Drawing for the job (mm, zero at the part's lowest x, y, z). Coordinates: 2 decimals unless noted, no trailing zeros. Loops run counter-clockwise (first coordinate to the right, second up) from the corner with the lowest first, then second, coordinate; pieces in that order, holes last. Notation, with made-up numbers: (-23, -39.5) - (25, -39.5) arc R15 cw to (25, -23.5) - close; hole circle Ø3 at (-2.5, -12). An arc over 180 degrees is marked (long way). One line per item, written item: value.
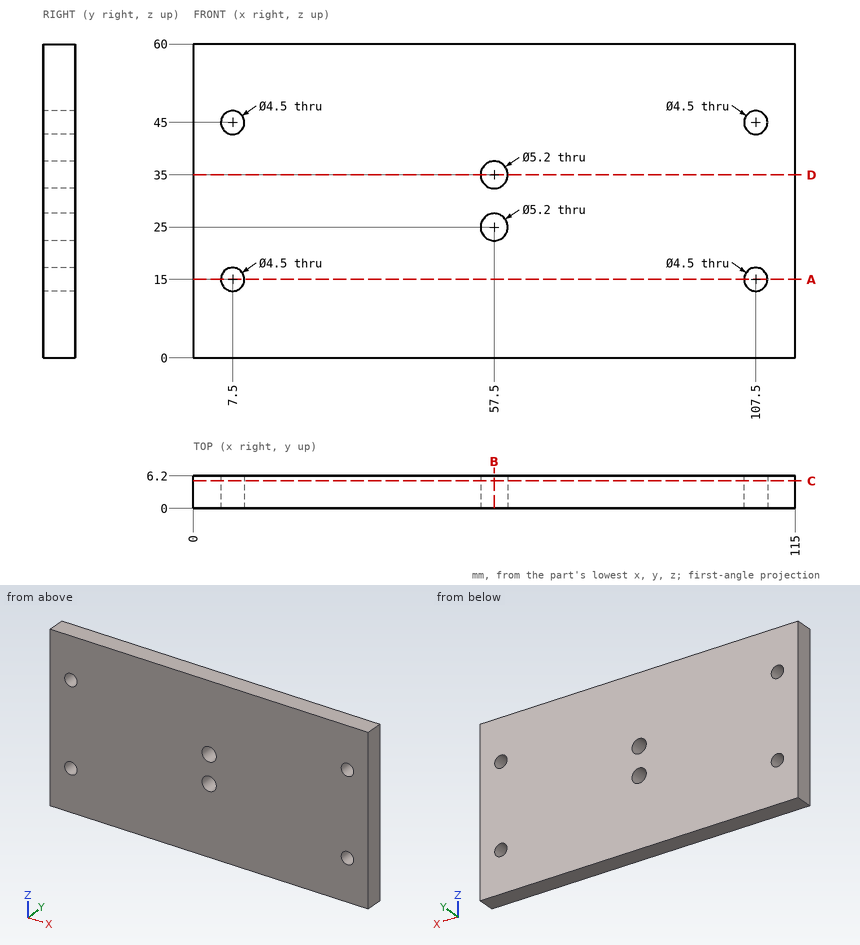
Item 1: Cut at C-C, the plane y = 5.25. Write the cut outline in (x, z), then the cut area to 3 significant figures.
Check result:
outline: (0, 0) - (115, 0) - (115, 60) - (0, 60) - close; hole circle Ø4.5 at (7.5, 15); hole circle Ø4.5 at (7.5, 45); hole circle Ø5.2 at (57.5, 25); hole circle Ø5.2 at (57.5, 35); hole circle Ø4.5 at (107.5, 15); hole circle Ø4.5 at (107.5, 45)
area: 6,790 mm^2
Item 2: Cut at A-A, the plane z = 15. Write the cut outline in (x, y).
Check result:
outline: (0, 0) - (5.25, 0) - (5.25, 6.2) - (0, 6.2) - close; (9.75, 0) - (105.25, 0) - (105.25, 6.2) - (9.75, 6.2) - close; (109.75, 0) - (115, 0) - (115, 6.2) - (109.75, 6.2) - close
Item 3: Cut at D-D, the plane z = 35. Write the cut outline in (x, y).
Check result:
outline: (0, 0) - (54.9, 0) - (54.9, 6.2) - (0, 6.2) - close; (60.1, 0) - (115, 0) - (115, 6.2) - (60.1, 6.2) - close
Item 4: Drop a flat-ended pin along its axis: P1, Ø4, axis at x = 7.5, z = 15, coming from the -Y side. Give the stop position or say it passes through.
Check result:
P1: passes through
Item 5: Probe probe 1 along Z at (x, y) = (107.5, 2); probe 2 along X at (y, z) = (3.5, 15); probe 3 along Z at (x, y) = (57.5, 3.75). List the from-to ranges inside material, lowest first. Write a range as from..to.
Check result:
probe 1: z = 0..12.75, 17.25..42.75, 47.25..60
probe 2: x = 0..5.25, 9.75..105.25, 109.75..115
probe 3: z = 0..22.4, 27.6..32.4, 37.6..60
Item 6: Cut at B-B, the plane x = 57.5. Write the cut outline in (y, z).
Check result:
outline: (0, 0) - (6.2, 0) - (6.2, 22.4) - (0, 22.4) - close; (0, 27.6) - (6.2, 27.6) - (6.2, 32.4) - (0, 32.4) - close; (0, 37.6) - (6.2, 37.6) - (6.2, 60) - (0, 60) - close
